Input: part model. Units: mm. Frame: model coordinates. A direction names the side the tool comes from. Round coordinates to 2 decimals unless told otherwise and drop trailing zeros. Write each loop counter-clockwise with the first axis right and the second up, starting at its lowest first coordinate (ties: lowest second). Pieces come first, ordered by that corner, then holes. Notation, with made-up numbers: M -12,84 L 12,84 A12 cw 12,105 Z; hole C 86,-15.5 d4. An arc over 180 degrees is marked long. Use one line per item in the form item = value. Start each with the question number.
```python
from build123d import *

# Parameters (mm, degrees)
SKETCH_1_W          = 50
SKETCH_1_H          = 50
EXTRUDE_1_DEPTH     = 12.5
FILLET_1_R          = 10
CUT_EXTRUDE_1_DEPTH = 6
SKETCH_3_R          = 3.375
CUT_EXTRUDE_2_DEPTH = 6
SKETCH_4_R          = 8.75
CUT_EXTRUDE_3_DEPTH = 3
SKETCH_5_W          = 67.74325056
SKETCH_5_H          = 59.124248938
SKETCH_5_R          = 12.5
CUT_EXTRUDE_4_DEPTH = 4.5
SKETCH_6_R          = 11.25
SKETCH_6_R_2        = 10.25
CUT_EXTRUDE_5_DEPTH = 2


with BuildPart() as part:
    # 草图1 → 凸台-拉伸1 (new body)
    with BuildSketch(Plane(origin=(0, 0, 0), x_dir=(1, 0, 0), z_dir=(0, 1, 0))):
        Rectangle(SKETCH_1_W, SKETCH_1_H)
    extrude(amount=EXTRUDE_1_DEPTH)

    # 圆角1
    fillet_1_edges = [part.edges().sort_by_distance(p)[0] for p in [
        (-25, 6.25, -25),
        (25, 6.25, -25),
        (25, 6.25, 25),
        (-25, 6.25, 25),
    ]]
    fillet(fillet_1_edges, radius=FILLET_1_R)

    # 草图2 → 切除-拉伸1 (cut)
    with BuildSketch(Plane(origin=(0, 12.5, 0), x_dir=(1, 0, 0), z_dir=(0, 1, 0))):
        with BuildLine():
            Line((3.5, 8.5), (3.5, -8.5))
            ThreePointArc((3.5, -8.5), (0, -12), (-3.5, -8.5))
            Line((-3.5, -8.5), (-3.5, 8.5))
            ThreePointArc((-3.5, 8.5), (0, 12), (3.5, 8.5))
        make_face()
    extrude(amount=-CUT_EXTRUDE_1_DEPTH, mode=Mode.SUBTRACT)

    # 草图3 → 切除-拉伸2 (cut)
    with BuildSketch(Plane(origin=(0, 6.5, 0), x_dir=(1, 0, 0), z_dir=(0, 1, 0))):
        with Locations(Location((0, -8.5, 0), (0, 0, 270))):
            Circle(SKETCH_3_R)
    extrude(amount=-CUT_EXTRUDE_2_DEPTH, mode=Mode.SUBTRACT)

    # 草图4 → 切除-拉伸3 (cut)
    with BuildSketch(Plane(origin=(0, 0, 0), x_dir=(-1, 0, 0), z_dir=(0, -1, 0))):
        with Locations(Location((0, -8.5, 0), (0, 0, 90))):
            Circle(SKETCH_4_R)
    extrude(amount=-CUT_EXTRUDE_3_DEPTH, mode=Mode.SUBTRACT)

    # 草图5 → 切除-拉伸4 (cut)
    with BuildSketch(Plane(origin=(0, 0, 0), x_dir=(-1, 0, 0), z_dir=(0, -1, 0))):
        with Locations((1.182484979, -0.052554888)):
            Rectangle(SKETCH_5_W, SKETCH_5_H)
        with Locations(Location((0, -8.5, 0), (0, 0, 90))):
            Circle(SKETCH_5_R, mode=Mode.SUBTRACT)
    extrude(amount=-CUT_EXTRUDE_4_DEPTH, mode=Mode.SUBTRACT)

    # 草图6 → 切除-拉伸5 (cut)
    with BuildSketch(Plane(origin=(0, 0, 0), x_dir=(-1, 0, 0), z_dir=(0, -1, 0))):
        with Locations(Location((0, -8.5, 0), (0, 0, 90))):
            Circle(SKETCH_6_R)
        with Locations(Location((0, -8.5, 0), (0, 0, 90))):
            Circle(SKETCH_6_R_2, mode=Mode.SUBTRACT)
    extrude(amount=-CUT_EXTRUDE_5_DEPTH, mode=Mode.SUBTRACT)


solid = part.part
```
Item 1: Ray query, line 1 (X direction, y = 0.75, z = 8.5); line 2 (X direction, y = 9, z = 8.5); line 3 (X direction, y = 5, z = 8.5) (3 decimals). Return the intervals inside material, ascending. Write a range as from..to.
Item 2: First-contact query: pin 1 (11 mm diameter, centred on x = 0, z = 8.5, fed in from -Y); pin 2 (4 mm diameter, centred on x = 15.5, z = 15.5, fed in from -Y); pin 3 (3 mm diameter, centred on y = 2.5, z = -11, fed in from +X); pin 4 (5.5 mm diameter, centred on x = -0.5, z = 3.5, fed in from +Y). Flat tips, straight axial feed; report the tip coordinate or a pass-through.
Item 3: Cut plane C-C (z = 6). Output: boundary loops of the cut face in (x, y).
Item 4: Draft query along X for faces 1 (the face through (0, 8, 25)), 2 (the face through (-22.15, 8.56, 21.99)), 3 (the face through (0.49, 0.99, 19.74)). Return one class per face: +X half, -X half, draft (parallel to the pull), parting line (faces both ways), or undercut.
Item 5: Cut plane B-B (x = 0). Output: boundary loops of the cut face in (y, z) (3 decimals).
Item 6: Cut plane D-D (y = 8.5). Output: boundary loops of the cut face in (x, z).
Item 7: Reachability of faces 4 (the face through (0, 10, 12)), 5 (the face through (-22.15, 8.56, -21.99)), 6 (the face through (0.55, 2.218, 20.988)) from +Z, -Z, +X, -X, +Y, -Y: full face, straight path, thin tool, end or side. Return the list, or none.
Item 8: Cut plane A-A (y = 1.25). Output: boundary loops of the cut face in (x, z), plus the area to 3 significant figures.
Final values:
q1.line_1 = -12.5..-11.25, -10.25..-8.75, 8.75..10.25, 11.25..12.5
q1.line_2 = -25..-3.5, 3.5..25
q1.line_3 = -25..-3.375, 3.375..25
q2.pin_1 = 3
q2.pin_2 = 4.5
q2.pin_3 = through
q2.pin_4 = 6.5
q3.outline = M -25,4.5 L -12.25,4.5 L -12.25,0 L -10.97,0 L -10.97,2 L -9.94,2 L -9.94,0 L -8.39,0 L -8.39,3 L -2.27,3 L -2.27,6.5 L -3.5,6.5 L -3.5,12.5 L -25,12.5 Z; M 2.27,3 L 8.39,3 L 8.39,0 L 9.94,0 L 9.94,2 L 10.97,2 L 10.97,0 L 12.25,0 L 12.25,4.5 L 25,4.5 L 25,12.5 L 3.5,12.5 L 3.5,6.5 L 2.27,6.5 Z
q4.face_1 = draft
q4.face_2 = -X half
q4.face_3 = undercut
q5.outline = M 0,-4 L 4.5,-4 L 4.5,-25 L 12.5,-25 L 12.5,-12 L 6.5,-12 L 6.5,5.125 L 3,5.125 L 3,-0.25 L 0,-0.25 L 0,-1.75 L 2,-1.75 L 2,-2.75 L 0,-2.75 Z; M 0,17.25 L 3,17.25 L 3,11.875 L 6.5,11.875 L 6.5,12 L 12.5,12 L 12.5,25 L 4.5,25 L 4.5,21 L 0,21 L 0,19.75 L 2,19.75 L 2,18.75 L 0,18.75 Z
q6.outline = M -25,-15 A10 ccw -15,-25 L 15,-25 A10 ccw 25,-15 L 25,15 A10 ccw 15,25 L -15,25 A10 ccw -25,15 Z; hole M -3.5,-8.5 A3.5 ccw 3.5,-8.5 L 3.5,8.5 A3.5 ccw -3.5,8.5 Z
q7.face_4 = +Y
q7.face_5 = -Z, -X, +Y, -Y
q7.face_6 = -Y
q8.outline = C 0,8.5 d25; C 0,8.5 d20.5; hole C 0,8.5 d22.5; hole C 0,8.5 d17.5
q8.area = 183 mm^2
